from build123d import *

# Parameters (mm, degrees)
BOSS_EXTRUDE1_DEPTH = 31.75
SKETCH19_W          = 15.860402013
SKETCH19_H          = 31.75
BOSS_EXTRUDE7_DEPTH = 2
SKETCH23_W          = 15.860402013
SKETCH23_H          = 2
BOSS_EXTRUDE8_DEPTH = 25
SKETCH24_R          = 1.27
CUT_EXTRUDE1_DEPTH  = 2.54


with BuildPart() as part:
    # Sketch2 → Boss-Extrude1 (new body)
    with BuildSketch(Plane.XY):
        with BuildLine():
            Line((-50.375618534, 45.609862895), (-50.351188886, 46.309436474))
            ThreePointArc((-50.351188886, 46.309436474), (-50.565618587, 46.88295476), (-51.12278195, 47.136868733))
            Line((-51.12278195, 47.136868733), (-55.780902554, 47.299533889))
            Line((-55.780902554, 47.299533889), (-47.850701548, 47.299533889))
            Line((-47.850701548, 47.299533889), (-47.850701548, 40.900752235))
            Line((-47.850701548, 40.900752235), (-48.952946324, 40.900752235))
            ThreePointArc((-48.952946324, 40.900752235), (-50.100996621, 41.129113637), (-51.074266668, 41.779431891))
            Line((-51.074266668, 41.779431891), (-53.375146928, 44.080312152))
            ThreePointArc((-53.375146928, 44.080312152), (-53.536830204, 44.931922499), (-52.803734096, 45.394471696))
            Line((-52.803734096, 45.394471696), (-50.685905631, 45.320515496))
            ThreePointArc((-50.685905631, 45.320515496), (-50.470836274, 45.400926634), (-50.375618534, 45.609862895))
        make_face()
    boss_extrude1 = extrude(amount=BOSS_EXTRUDE1_DEPTH)

    # Mirror2: Boss-Extrude1 across plane
    add(boss_extrude1.mirror(Plane(origin=(-47.850701548, 40.900752235, 31.75), x_dir=(0, 0, 1), z_dir=(-1, 0, 0))))

    # Sketch19 → Boss-Extrude7 (add)
    with BuildSketch(Plane(origin=(0, 47.299533889, 0), x_dir=(1, 0, 0), z_dir=(0, 1, 0))):
        with Locations((-47.850701548, -15.875)):
            Rectangle(SKETCH19_W, SKETCH19_H)
    extrude(amount=BOSS_EXTRUDE7_DEPTH)

    # Sketch23 → Boss-Extrude8 (add)
    with BuildSketch(Plane(origin=(0, 49.299533889, 0), x_dir=(1, 0, 0), z_dir=(0, 1, 0))):
        with Locations((-47.850701548, -30.75)):
            Rectangle(SKETCH23_W, SKETCH23_H)
    extrude(amount=BOSS_EXTRUDE8_DEPTH)

    # Sketch24 → Cut-Extrude1 (cut)
    with BuildSketch(Plane(origin=(0, 0, 29.75), x_dir=(-1, 0, 0), z_dir=(0, 0, -1))):
        with Locations((47.850701548, 67.949533889)):
            Circle(SKETCH24_R)
    extrude(amount=-CUT_EXTRUDE1_DEPTH, mode=Mode.SUBTRACT)


solid = part.part
The listing builds one solid part. Answer for the finished solid, in the listing's coordinates (mm). A direction names the side the tool comes from. Give positions to 0.01 mm unless a question says otherwise; leave off trailing zeros. Write each loop counter-clockwise with the first axis right and the second up, starting at its lowest first coordinate (ties: lowest second). Pieces come first, ordered by that corner, then holes.
Item 1: Which of the six approach directions +Z, -Z, +X, -X, +Y, -Y give full straight-line access (tool end or side, diameter ignored) to faces 1 (the cylindrical face through (-45, 47, 16)), 2 (the cylindrical face through (-50.56, 46.876, 15.653)), 3 (the flat face through (-48, 49.3, 15))?
Item 2: Section B-B, the plane z = 3.5 is taken. Write down the section's boundary in (x, y), plus the area to 3 significant figures.
Item 3: Determine the mould class of faces 4 (the cylindrical face through (-53.54, 44.92, 15.65)), 5 (the flat face through (-48, 74.3, 31)), 6 (the cylindrical face through (-45.62, 41.12, 15.65)), 7 (the flat face through (-48, 62, 29.75)) for opening direction Y: released by +Y, released by -Y, zero draft, split by the parting line, or undercut.
Item 4: Find the intervals of material crossed by line 1 along Z through (x, y) = (-48.5, 57); line 2 along Y through (x, z) = (-47.25, 26); line 3 along Y through (x, z) = (-53.5, 6), in increasing order.
Item 5: Section A-A, the plane x = -48 is taken. Write down the section's boundary in (y, z).
Item 6: Section D-D, the plane x = -54.25 is taken. Write down the section's boundary in (y, z), plus the area to 3 significant figures.
Item 7: Flat-ended cylindrical pins translate along their axes: P1, Ø1, axis at x = -44, z = 27.5, coming from the +Y side; P2, Ø3, axis at x = -42, y = 53.5, coming from the -Z side; P3, Ø3, axis at x = -47.85, y = 67.95, coming from the +Z side; P4, Ø3, axis at y = 52.5, z = 14.5, coming from the -X side. Find the tip coordinate at first contact, or state that the pin passes through.
Item 8: Section C-C, the plane y = 51 is taken. Write down the section's boundary in (x, z), plus the area to 3 significant figures.
Completed:
1. face 1: +Z, -Z, +X
1. face 2: +Z, -Z, -X
1. face 3: -Z, +X, -X, +Y
2. outline: (-55.78, 47.3) - (-51.12, 47.14) arc R0.8 cw to (-50.35, 46.31) - (-50.38, 45.61) arc R0.3 cw to (-50.69, 45.32) - (-52.8, 45.39) arc R0.77 ccw to (-53.38, 44.08) - (-51.07, 41.78) arc R3 ccw to (-48.95, 40.9) - (-46.75, 40.9) arc R3 ccw to (-44.63, 41.78) - (-42.33, 44.08) arc R0.77 ccw to (-42.9, 45.39) - (-45.02, 45.32) arc R0.3 cw to (-45.33, 45.61) - (-45.35, 46.31) arc R0.8 cw to (-44.58, 47.14) - (-39.92, 47.3) - (-39.92, 49.3) - (-55.78, 49.3) - close
2. area: 81.8 mm2
3. face 4: undercut
3. face 5: released by +Y
3. face 6: released by -Y
3. face 7: zero draft
4. line 1: z = 29.75 to 31.75
4. line 2: y = 40.9 to 49.3
4. line 3: y = 44.24 to 45.01, 47.22 to 49.3
5. outline: (40.9, 0) - (49.3, 0) - (49.3, 29.75) - (66.69, 29.75) - (66.69, 31.75) - (40.9, 31.75) - close; (69.21, 29.75) - (74.3, 29.75) - (74.3, 31.75) - (69.21, 31.75) - close
6. outline: (47.25, 0) - (49.3, 0) - (49.3, 29.75) - (74.3, 29.75) - (74.3, 31.75) - (47.25, 31.75) - close
6. area: 115 mm2
7. P1: stops at y = 49.3
7. P2: stops at z = 29.75
7. P3: stops at z = 31.75
7. P4: passes through
8. outline: (-55.78, 29.75) - (-39.92, 29.75) - (-39.92, 31.75) - (-55.78, 31.75) - close
8. area: 31.7 mm2
